Here's how the part is built. I have some questions about the finished solid (model axes, mm). A direction names the side the tool comes from. Give positions to 0.01 mm unless a question says otherwise; leave off trailing zeros. Loops run counter-clockwise (first coordinate to the right, second up) from the corner with the lowest first, then second, coordinate; pieces in that order, holes last. Notation, with made-up numbers: (-22, 0) - (18, 0) arc R28 cw to (18, 34) - close; hole circle Ø10 at (-31.5, -30.5). An arc over 180 degrees is marked (long way). One line per item, written item: value. Start each with the question number.
```python
from build123d import *

# Parameters (mm, degrees)
SKETCH1_R           = 160.3375
SKETCH1_R_2         = 8.3
BOSS_EXTRUDE1_DEPTH = 2.85
CUT_EXTRUDE1_DEPTH  = 227.769376928


with BuildPart() as part:
    # Sketch1 → Boss-Extrude1 (new body)
    with BuildSketch(Plane(origin=(0, 0, 0), x_dir=(1, 0, 0), z_dir=(0, 1, 0))):
        with Locations(Location((0, 0, 0), (0, 0, 270))):
            Circle(SKETCH1_R)
        with Locations(Location((0, 0, 0), (0, 0, 270))):
            Circle(SKETCH1_R_2, mode=Mode.SUBTRACT)
    extrude(amount=BOSS_EXTRUDE1_DEPTH)

    # Sketch3 → Cut-Extrude1 (cut, through all)
    with BuildSketch(Plane(origin=(0, 2.85, 0), x_dir=(1, 0, 0), z_dir=(0, 1, 0))):
        Polygon((-15, 10), (-106.923881554, 101.923881554), (-145, 10), align=None)
        Polygon((-95.45941546, 109.601551084), (-3.535533906, 17.67766953), (-3.535533906, 147.67766953), align=None)
        Polygon((10, 145), (10, 15), (101.923881554, 106.923881554), align=None)
        Polygon((109.601551084, 95.45941546), (17.67766953, 3.535533906), (147.67766953, 3.535533906), align=None)
        Polygon((145, -10), (15, -10), (106.923881554, -101.923881554), align=None)
        Polygon((95.45941546, -109.601551084), (3.535533906, -17.67766953), (3.535533906, -147.67766953), align=None)
        Polygon((-10, -145), (-10, -15), (-101.923881554, -106.923881554), align=None)
        Polygon((-109.601551084, -95.45941546), (-17.67766953, -3.535533906), (-147.67766953, -3.535533906), align=None)
    extrude(amount=-CUT_EXTRUDE1_DEPTH, mode=Mode.SUBTRACT)


solid = part.part
```
(1) If we section it at A-A on y = 0.6: Give the number of separate pieces and of enclosed holes in the cut face, plus the area to 3 significant figures.
(2) Will these pins go through, and if not, where does the flat tip stop? pin 1 (0.9 mm diameter, centred on y = 1, z = 101.5, fed in from +X); pin 2 (1.4 mm diameter, centred on x = -57, y = 1, fed in from +Z); pin 3 (1.5 mm diameter, centred on x = -31.5, y = 2.5, fed in from -Z).
(3) For faces 1 (the face through (-125.695, 1.445, -56.605)), 2 (the face through (-33, 2.85, -2)), which set-ups out of +Z, -Z, +X, -X, +Y, -Y let a thin tool reach every point of the face, with its end or its side?
(4) If we section it at C-C on x = 80: List the corners of the cut face in (y, z) for me.
(5) Please list where these lines run through material, in increasing order: probe 1 along X at (y, z) = (1.2, 0); probe 2 along X at (y, z) = (1.95, 11); probe 3 along X at (y, z) = (1.6, 136). Write a range as from..to.
(6) If we section it at B-B on z = -44: List the corners of the cut face in (x, y) for me.
(7) If we mould it in two halves opening along X, with no side actions, what happens to faces 3 (the face through (-33, 0, -2)), 4 (the face through (7.05, 1.405, -160.182)), 5 (the face through (-50.14, 1.44, -64.28))? For each: pulls with the +X half, pulls with the -X half, needs draft (parallel to the pull), parting line crosses it, or undercut.
Found:
1. separate pieces: 1
1. enclosed holes: 9
1. area: 32,700 mm^2
2. pin 1: x = 124.49
2. pin 2: z = 150.13
2. pin 3: z = -157.36
3. face 1: +Y, -Y
3. face 2: +Z, -Z, +X, -X, +Y
4. outline: (0, -138.95) - (2.85, -138.95) - (2.85, -116.01) - (0, -116.01) - close; (0, -85) - (2.85, -85) - (2.85, -65.86) - (0, -65.86) - close; (0, -3.54) - (2.85, -3.54) - (2.85, 10) - (0, 10) - close; (0, 75) - (2.85, 75) - (2.85, 94.14) - (0, 94.14) - close; (0, 116.01) - (2.85, 116.01) - (2.85, 138.95) - (0, 138.95) - close
5. probe 1: -160.34..-8.3, 8.3..160.34
5. probe 2: -159.96..-144.59, -25.14..16, 144.59..159.96
5. probe 3: -84.92..-31.73, -10..3.54, 31.73..84.92
6. outline: (-154.18, 0) - (-130.92, 0) - (-130.92, 2.85) - (-154.18, 2.85) - close; (-49, 0) - (-29.86, 0) - (-29.86, 2.85) - (-49, 2.85) - close; (-3.54, 0) - (10, 0) - (10, 2.85) - (-3.54, 2.85) - close; (39, 0) - (58.14, 0) - (58.14, 2.85) - (39, 2.85) - close; (130.92, 0) - (154.18, 0) - (154.18, 2.85) - (130.92, 2.85) - close
7. face 3: needs draft
7. face 4: parting line crosses it
7. face 5: undercut
